Model file for the job. Use its own axes, mm. A direction names the side the tool comes from. Give positions to 0.01 mm unless a question says otherwise; leave off trailing zeros. Order: outer loops, then holes, each group sorted by start corner. A loop starts at its lowest first (then second) coordinate and runs counter-clockwise, first axis right, second up. Notation, with made-up numbers: (63, 44.5) -> (111, 44.5) arc R24 cw to (111, 60.5) -> close; hole circle Ø11 at (-38, 60.5). An arc over 180 degrees is marked (long way). Use CSV: the item, a comma, the result in double quotes. Start each with the question number.
1. Cut at A-A on y = -7. List the corners of the cut face in (x, z).
2. Drop flat-ended pins along their axis: pin 1 (6 mm diameter, centred on x = 4, y = -5.5, fed in from +Z); pin 2 (3 mm diameter, centred on x = 2.5, z = 2.5, fed in from -Y); pin 3 (2 mm diameter, centred on x = -3, y = -4.5, fed in from -Z); pin 4 (4 mm diameter, centred on x = -3, y = -1.5, fed in from -Z). Give the stop position or say it passes through.
3. Wall check: line 1 (Y direction, x = 1.75, z = 4.25); line 2 (Y direction, x = -1.25, z = 3); line 3 (Z direction, x = 3.5, y = 0.5). Give the ranges that are in metal, low to high. Write a range as from..to.
4. 3-axis set-ups, long thin cutter, end or side, ignore diameter. For faces 1 (the cylindrical face through (-0.189, 0.751, 5.356)), 2 (the cylindrical face through (-0.83, -4.57, -3.72)): which of +Z, -Z, +X, -X, +Y, -Y reach the whole face in a straight line?
```python
from build123d import *

# Parameters (mm, degrees)
F0_R     = 3.81
F1_DEPTH = 12.7
F2_R     = 3.429
F4_DEPTH = 1.524


with BuildPart() as f1:
    # F0 (on Front) → F1 (new body)
    with BuildSketch(Plane.XZ):
        Circle(F0_R)
    extrude(amount=F1_DEPTH)

    # F2
    f2_edges = [f1.edges().sort_by_distance(p)[0] for p in [
        (-3.81, -12.7, 0),
    ]]
    fillet(f2_edges, radius=F2_R)

    # F3 (on face) → F4 (join)
    with BuildSketch(Plane(origin=(0, 0, 0), x_dir=(-1, 0, 0), z_dir=(0, 1, 0))):
        with BuildLine():
            Line((-3.101973, -4.370782), (3.101973, -4.370782))
            ThreePointArc((3.101973, -4.370782), (0, 5.359661), (-3.101973, -4.370782))
        make_face()
    extrude(amount=F4_DEPTH)


solid = f1.part
```
Verdict:
1,outline,"circle Ø7.62 at (0, 0)"
2,pin 1,"z = 3.68"
2,pin 2,"y = -12.27"
2,pin 3,"z = -3.24"
2,pin 4,"z = -4.37"
3,line 1,"0..1.52"
3,line 2,"-11.15..1.52"
3,line 3,"-4.06..4.06"
4,face 1,"+Y, -Y"
4,face 2,"-Y"
